For this review, take the finished solid that the model builds, in its own axes (mm). Face numbers are marked on the shaded views. A direction names the side the tool comes from. Give positions to 0.01 mm unless a question says otherwise; leave off trailing zeros. Write each loop counter-clockwise with the first axis right and the second up, starting at its lowest first coordinate (ties: lowest second). Pieces come first, ordered by that corner, then holes. Notation, with made-up numbers: (0, -33.5) -> (24, -33.5) arc R23 ccw to (24, -7.5) -> close; hole circle Ø8 at (58.5, 2). An arc over 180 degrees is marked (long way). Return JSON: item names as keys, results as strings.
from build123d import *

# Parameters (mm, degrees)
SKETCH1_R           = 39.5
BOSS_EXTRUDE1_DEPTH = 153.67
CUT_EXTRUDE1_START  = -5
CUT_EXTRUDE1_DEPTH  = 5
SKETCH4_5_R         = 9
BOSS_EXTRUDE2_DEPTH = 6
BOSS_EXTRUDE3_DEPTH = 18
SKETCH4_7_R         = 3.3
CUT_EXTRUDE3_DEPTH  = 17
BOSS_EXTRUDE4_DEPTH = 4
CUT_EXTRUDE5_DEPTH  = 1
SKETCH9_R           = 6.042977367
CUT_EXTRUDE6_DEPTH  = 10
CIRPATTERN1_COUNT   = 8
SKETCH9_3_R         = 10.665128642
CUT_EXTRUDE7_DEPTH  = 10
BOSS_EXTRUDE5_START = 9
SKETCH10_R          = 8
BOSS_EXTRUDE5_DEPTH = 9
FILLET3_R           = 0.5
FILLET4_R           = 1


with BuildPart() as part:
    # Sketch1 → Boss-Extrude1 (new body)
    with BuildSketch(Plane(origin=(0, 0, 0), x_dir=(1, 0, 0), z_dir=(0, 1, 0))):
        with Locations(Location((0, 0, 0), (0, 0, 270))):
            Circle(SKETCH1_R)
    extrude(amount=BOSS_EXTRUDE1_DEPTH)

    # Sketch2 → Revolve1 (revolve)
    with BuildSketch(Plane.XY, mode=Mode.PRIVATE) as revolve1_sk:
        Polygon((0, 153.67), (-39.5, 153.67), (-32, 158.67), (0, 158.67), align=None)
    revolve(revolve1_sk.sketch.rotate(Axis((0, 158.67, 0), (0, -1, 0)), 270), axis=Axis((0, 158.67, 0), (0, -1, 0)))

    # Sketch4 → Cut-Extrude1 (cut)
    with BuildSketch(Plane(origin=(0, 158.67, 0), x_dir=(1, 0, 0), z_dir=(0, 1, 0)).offset(CUT_EXTRUDE1_START)):
        with BuildLine():
            Line((-39.017846302, 6.152858683), (-28.858540725, 6.152858683))
            ThreePointArc((-28.858540725, 6.152858683), (-22.705682042, 0), (-28.858540725, -6.152858683))
            Line((-28.858540725, -6.152858683), (-39.017846302, -6.152858683))
            ThreePointArc((-39.017846302, -6.152858683), (-39.5, 0), (-39.017846302, 6.152858683))
        make_face()
        with BuildLine():
            Line((-6.152858683, 39.017846302), (-6.152858683, 28.858540725))
            ThreePointArc((-6.152858683, 28.858540725), (0, 22.705682042), (6.152858683, 28.858540725))
            Line((6.152858683, 28.858540725), (6.152858683, 39.017846302))
            ThreePointArc((6.152858683, 39.017846302), (0, 39.5), (-6.152858683, 39.017846302))
        make_face()
        with BuildLine():
            Line((39.017846302, 6.152858683), (28.858540725, 6.152858683))
            ThreePointArc((28.858540725, 6.152858683), (22.705682042, 0), (28.858540725, -6.152858683))
            Line((28.858540725, -6.152858683), (39.017846302, -6.152858683))
            ThreePointArc((39.017846302, -6.152858683), (39.5, 0), (39.017846302, 6.152858683))
        make_face()
        with BuildLine():
            Line((6.152858683, -39.017846302), (6.152858683, -28.858540725))
            ThreePointArc((6.152858683, -28.858540725), (0, -22.705682042), (-6.152858683, -28.858540725))
            Line((-6.152858683, -28.858540725), (-6.152858683, -39.017846302))
            ThreePointArc((-6.152858683, -39.017846302), (0, -39.5), (6.152858683, -39.017846302))
        make_face()
    extrude(amount=CUT_EXTRUDE1_DEPTH, mode=Mode.SUBTRACT)

    # Sketch4<5> → Boss-Extrude2 (add)
    with BuildSketch(Plane(origin=(0, 158.67, 0), x_dir=(1, 0, 0), z_dir=(0, 1, 0))):
        with Locations(Location((0, 0, 0), (0, 0, 270))):
            Circle(SKETCH4_5_R)
    extrude(amount=BOSS_EXTRUDE2_DEPTH)

    # Sketch5 → Boss-Extrude3 (add)
    with BuildSketch(Plane(origin=(0, 164.67, 0), x_dir=(1, 0, 0), z_dir=(0, 1, 0))):
        with BuildLine():
            Line((6.156533816, 5.108531235), (6.156533816, -5.108531235))
            ThreePointArc((6.156533816, -5.108531235), (-8, 0), (6.156533816, 5.108531235))
        make_face()
    extrude(amount=BOSS_EXTRUDE3_DEPTH)

    # Sketch4<7> → Cut-Extrude3 (cut)
    with BuildSketch(Plane(origin=(0, 158.67, 0), x_dir=(1, 0, 0), z_dir=(0, 1, 0))):
        with Locations(Location((12.5, 12.5, 0), (0, 0, 270))):
            Circle(SKETCH4_7_R)
        with Locations(Location((-12.5, 12.5, 0), (0, 0, 90))):
            Circle(SKETCH4_7_R)
        with Locations(Location((12.5, -12.5, 0), (0, 0, 90))):
            Circle(SKETCH4_7_R)
        with Locations(Location((-12.5, -12.5, 0), (0, 0, 270))):
            Circle(SKETCH4_7_R)
    extrude(amount=-CUT_EXTRUDE3_DEPTH, mode=Mode.SUBTRACT)

    # Sketch6 → Boss-Extrude4 (add)
    with BuildSketch(Plane(origin=(0, 153.67, 0), x_dir=(1, 0, 0), z_dir=(0, 1, 0))):
        Polygon((1.905255888, -30.661808974), (-1.905255888, -30.661808974), (-3.810511777, -33.961808974), (-1.905255888, -37.261808974), (1.905255888, -37.261808974), (3.810511777, -33.961808974), align=None)
        Polygon((-37.261808974, 1.905255888), (-37.261808974, -1.905255888), (-33.961808974, -3.810511777), (-30.661808974, -1.905255888), (-30.661808974, 1.905255888), (-33.961808974, 3.810511777), align=None)
        Polygon((1.905255888, 37.261808974), (-1.905255888, 37.261808974), (-3.810511777, 33.961808974), (-1.905255888, 30.661808974), (1.905255888, 30.661808974), (3.810511777, 33.961808974), align=None)
        Polygon((37.261808974, -1.905255888), (37.261808974, 1.905255888), (33.961808974, 3.810511777), (30.661808974, 1.905255888), (30.661808974, -1.905255888), (33.961808974, -3.810511777), align=None)
    extrude(amount=BOSS_EXTRUDE4_DEPTH)

    # Sketch8 → Cut-Extrude5 (cut)
    with BuildSketch(Plane(origin=(0, 157.67, 0), x_dir=(1, 0, 0), z_dir=(0, 1, 0))):
        Polygon((-35.761808974, 1.039230485), (-35.761808974, -1.039230485), (-33.961808974, -2.078460969), (-32.161808974, -1.039230485), (-32.161808974, 1.039230485), (-33.961808974, 2.078460969), align=None)
        Polygon((-1.039230485, -35.761808974), (1.039230485, -35.761808974), (2.078460969, -33.961808974), (1.039230485, -32.161808974), (-1.039230485, -32.161808974), (-2.078460969, -33.961808974), align=None)
        Polygon((1.039230485, 35.761808974), (-1.039230485, 35.761808974), (-2.078460969, 33.961808974), (-1.039230485, 32.161808974), (1.039230485, 32.161808974), (2.078460969, 33.961808974), align=None)
        Polygon((35.761808974, -1.039230485), (35.761808974, 1.039230485), (33.961808974, 2.078460969), (32.161808974, 1.039230485), (32.161808974, -1.039230485), (33.961808974, -2.078460969), align=None)
    extrude(amount=-CUT_EXTRUDE5_DEPTH, mode=Mode.SUBTRACT)

    # Sketch9 → Cut-Extrude6 (cut)
    with BuildSketch(Plane.XZ):
        with Locations(Location((22.400920741, -0.076389237, 0), (0, 0, 270))):
            Circle(SKETCH9_R)
    cut_extrude6 = extrude(amount=-CUT_EXTRUDE6_DEPTH, mode=Mode.SUBTRACT)

    # CirPattern1: Cut-Extrude6 ×8 about axis
    cirpattern1_axis = Axis((-0.536857588, 0, 0.001830735), (0, 1, 0))
    for i in range(1, CIRPATTERN1_COUNT):
        add(cut_extrude6.rotate(cirpattern1_axis, i * 360 / CIRPATTERN1_COUNT), mode=Mode.SUBTRACT)

    # Sketch9<3> → Cut-Extrude7 (cut)
    with BuildSketch(Plane.XZ):
        with Locations(Location((0, 0, 0), (0, 0, 270))):
            Circle(SKETCH9_3_R)
    extrude(amount=-CUT_EXTRUDE7_DEPTH, mode=Mode.SUBTRACT)

    # Sketch10 → Boss-Extrude5 (add)
    with BuildSketch(Plane.XZ.offset(-10).offset(BOSS_EXTRUDE5_START)):
        with Locations(Location((0, 0, 0), (0, 0, 270))):
            Circle(SKETCH10_R)
    extrude(amount=-BOSS_EXTRUDE5_DEPTH)

    # Fillet3
    fillet3_edges = [part.edges().sort_by_distance(p)[0] for p in [
        (0, 1, 8),
    ]]
    fillet(fillet3_edges, radius=FILLET3_R)

    # Fillet4
    fillet4_edges = [part.edges().sort_by_distance(p)[0] for p in [
        (6.156533816, 182.67, 0),
        (-8, 182.67, 0),
    ]]
    fillet(fillet4_edges, radius=FILLET4_R)


solid = part.part
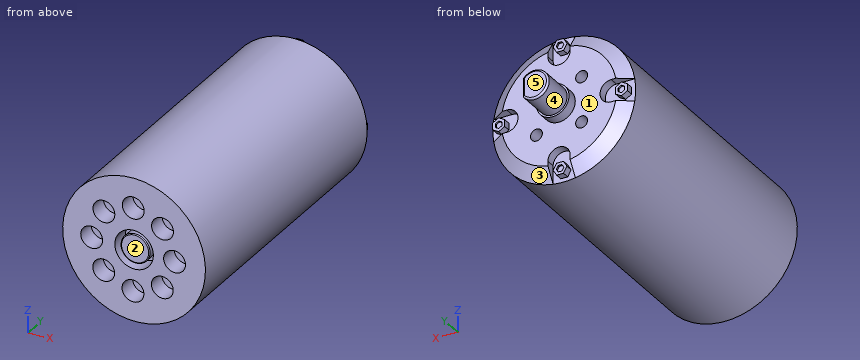
1. For the marked faces 4 and 5, list the 3-axis set-ups (+Z, -Z, +X, -X, +Y, -Y) from which the entire face can be reached by the end or side of a thin tool; tool diameter is ignored.
Results found:
{"face 4": "+Y", "face 5": "+Z, -Z, +X, -X, +Y"}
2. The part is to be moulded in two halves that separate along X. For the marked faces 1, 2 and 3, say which applies: +X half, -X half, draft (parallel to the pull), parting line (faces both ways), or undercut.
Results found:
{"face 1": "draft", "face 2": "undercut", "face 3": "+X half"}
3. To check wall thickness, follow probe 1 along Z at (x, y) = (-12, 148); probe 2 along Z at (x, y) = (11, 146.5); probe 3 along X at (y, z) = (146, -12.5). State the ranges of each line that lie inside material, in increasing order.
Results found:
{"probe 1": "z = -37.63 to -15.76, -9.24 to 9.24, 15.76 to 37.63", "probe 2": "z = -37.94 to -15.44, -9.56 to 9.56, 15.44 to 37.94", "probe 3": "x = -37.47 to -15.8, -9.2 to 9.2, 15.8 to 37.47"}
4. Add section A-A, the plane y = 149. State the section outline as (x, z) points, plus the area to 3 significant figures.
Results found:
{"outline": "circle Ø79 at (0, 0); hole circle Ø6.6 at (-12.5, -12.5); hole circle Ø6.6 at (-12.5, 12.5); hole circle Ø6.6 at (12.5, -12.5); hole circle Ø6.6 at (12.5, 12.5)", "area": "4,760 mm²"}
5. Add section B-B, the plane y = 116. State the section outline as (x, z) points.
Results found:
{"outline": "circle Ø79 at (0, 0)"}
6. For pin 1 (13.5 mm diameter, centred on x = -15.5, z = 14, fed in from -Y); pin 2 (0.5 mm diameter, centred on y = 157.5, z = 0.5, fed in from -X); pin 3 (12 mm diameter, centred on x = 21.5, y = 66, fed in from +Z); pin 4 (1.5 mm diameter, centred on y = 103, z = 26, fed in from -X), all flat-tipped, find the tip position at first contact; note any pin that passes through.
Results found:
{"pin 1": "stops at y = 0", "pin 2": "stops at x = -37.26", "pin 3": "stops at z = 36.33", "pin 4": "stops at x = -30.38"}
